Build history of the part. All positions in model axes, mm. Face numbers are marked on the shaded views. A direction names the side the tool comes from. Coordinates: 2 decimals unless noted, no trailing zeros. Order: outer loops, then holes, each group sorted by start corner. A loop starts at its lowest first (then second) coordinate and runs counter-clockwise, first axis right, second up. Notation, with made-up numbers: M -32.75,87 L -7.75,87 A15 ccw -7.75,100 Z; hole C 10.25,59.5 d7. An arc over 180 degrees is marked long. Use a Markdown table: item, result. Add a question column.
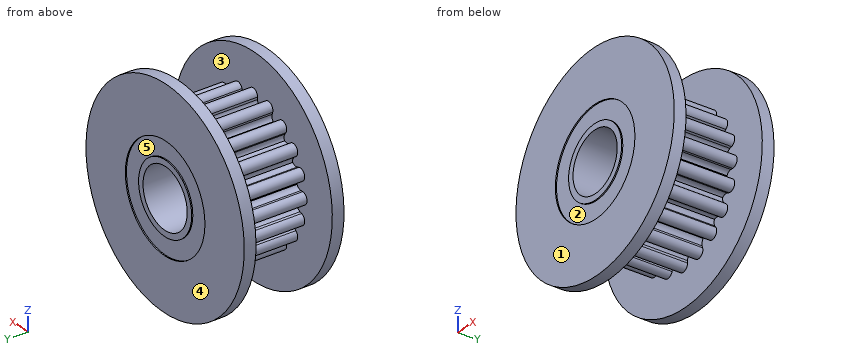
from build123d import *

# Parameters (mm, degrees)
SKETCH1_R           = 8.95
SKETCH1_R_2         = 2.5
BOSS_EXTRUDE1_DEPTH = 1
SKETCH2_R           = 5
SKETCH2_R_2         = 2.5
BOSS_EXTRUDE2_DEPTH = 3.25
BOSS_EXTRUDE3_DEPTH = 3.25
CIRPATTERN1_COUNT   = 20
SKETCH4_R           = 4.5
SKETCH4_R_2         = 3
CUT_EXTRUDE1_DEPTH  = 0.1


with BuildPart() as part:
    # Sketch1 → Boss-Extrude1 (new body)
    with BuildSketch(Plane(origin=(0, 0, 0), x_dir=(1, 0, 0), z_dir=(0, 1, 0))):
        with Locations(Location((0, 0, 0), (0, 0, 270))):
            Circle(SKETCH1_R)
        with Locations(Location((0, 0, 0), (0, 0, 270))):
            Circle(SKETCH1_R_2, mode=Mode.SUBTRACT)
    extrude(amount=BOSS_EXTRUDE1_DEPTH)

    # Sketch2 → Boss-Extrude2 (add)
    with BuildSketch(Plane(origin=(0, 1, 0), x_dir=(1, 0, 0), z_dir=(0, 1, 0))):
        with Locations(Location((0, 0, 0), (0, 0, 90))):
            Circle(SKETCH2_R)
        with Locations(Location((0, 0, 0), (0, 0, 270))):
            Circle(SKETCH2_R_2, mode=Mode.SUBTRACT)
    extrude(amount=BOSS_EXTRUDE2_DEPTH)

    # Sketch3 → Boss-Extrude3 (add)
    with BuildSketch(Plane(origin=(0, 1, 0), x_dir=(1, 0, 0), z_dir=(0, 1, 0))):
        with BuildLine():
            Line((0.5, 5.6), (0.5, 5.408326913))
            ThreePointArc((0.5, 5.408326913), (0.615646943, 5.088525839), (0.909090909, 4.91666083))
            Line((0.909090909, 4.91666083), (-0.909090909, 4.91666083))
            ThreePointArc((-0.909090909, 4.91666083), (-0.615646943, 5.088525839), (-0.5, 5.408326913))
            Line((-0.5, 5.408326913), (-0.5, 5.6))
            ThreePointArc((-0.5, 5.6), (0, 6.1), (0.5, 5.6))
        make_face()
    boss_extrude3 = extrude(amount=BOSS_EXTRUDE3_DEPTH)

    # CirPattern1: Boss-Extrude3 ×20 about axis
    cirpattern1_axis = Axis((0, 0, 0), (0, 1, 0))
    for i in range(1, CIRPATTERN1_COUNT):
        add(boss_extrude3.rotate(cirpattern1_axis, i * 360 / CIRPATTERN1_COUNT))

    # Sketch4 → Cut-Extrude1 (cut)
    with BuildSketch(Plane.XZ):
        with Locations(Location((0, 0, 0), (0, 0, 270))):
            Circle(SKETCH4_R)
        with Locations(Location((0, 0, 0), (0, 0, 270))):
            Circle(SKETCH4_R_2, mode=Mode.SUBTRACT)
    extrude(amount=-CUT_EXTRUDE1_DEPTH, mode=Mode.SUBTRACT)

    # Mirror1: part across plane


with BuildPart() as part_1:
    add(part.part)
    add(part.part.mirror(Plane.ZX.offset(4.25)))


solid = part_1.part
(1) Slice it at D-D on x = 7.75. Give the cut face in (y, z), and give its area (3 significant figures).
(2) Slice it at C-C on x = -7. Give the cut face in (y, z), and give its area (3 significant figures).
(3) Mould opens along X. For the marked faces 1 and 2 say: released by +X, released by -X, zero draft, split by the parting line, or undercut.
(4) Drop flat-ended pins along their axis: P1, Ø7, axis at x = 0, z = 0, coming from the -Y side; P2, Ø1, axis at x = -1, y = 6, coming from the +Z side; P3, Ø4, axis at x = 3.5, y = 6.5, coming from the +Z side; P4, Ø1, axis at x = -0.5, z = 1.5, coming from the -Y side. Give the stop position or say it passes through.
(5) Which spindle directions (+Z, -Z, +X, -X, +Y, -Y) get a long thin tool onto all of the face, cutting with end or side? Do the marked faces 3, 4 and 5. Say none if no direction does.
(6) Drill centre lines: line 1 along Y through (x, z) = (-6.25, 0.5); line 2 along Y through (x, z) = (-4, -2); line 3 along X through (y, z) = (2.5, -5.5). Where is each one in solid material? Low to high. Write a range as from..to.
Solutions:
| question | item | result |
|---|---|---|
| 1 | outline | M 0,-4.48 L 1,-4.48 L 1,4.48 L 0,4.48 Z; M 7.5,-4.48 L 8.5,-4.48 L 8.5,4.48 L 7.5,4.48 Z |
| 1 | area | 17.9 mm² |
| 2 | outline | M 0,-5.58 L 1,-5.58 L 1,5.58 L 0,5.58 Z; M 7.5,-5.58 L 8.5,-5.58 L 8.5,5.58 L 7.5,5.58 Z |
| 2 | area | 22.3 mm² |
| 3 | face 1 | zero draft |
| 3 | face 2 | undercut |
| 4 | P1 | y = 0 |
| 4 | P2 | z = 5.77 |
| 4 | P3 | z = 8.77 |
| 4 | P4 | through |
| 5 | face 3 | none |
| 5 | face 4 | +Z, -Z, +X, -X, +Y |
| 5 | face 5 | +Y |
| 6 | line 1 | 0..1, 7.5..8.5 |
| 6 | line 2 | 0.1..8.4 |
| 6 | line 3 | -2.2..-1.26, -0.5..0.5, 1.26..2.2 |
